from build123d import *

# Parameters (mm, degrees)
F2_SIZE  = 0.79375
F3_R     = 11.1125
F4_DEPTH = 2.3622


with BuildPart() as f1:
    # F0 (on Right) → F1 (revolve)
    with BuildSketch(Plane.YZ):
        Polygon((0, 12.7), (0, 0), (19.05, 0), (19.05, 6.35), (13.396951, 6.35), (5.807927, 12.7), align=None)
    revolve(axis=Axis((0, 9.525, 0), (0, -1, 0)))

    # F2
    f2_edges = [f1.edges().sort_by_distance(p)[0] for p in [
        (0, 0, -12.7),
    ]]
    chamfer(f2_edges, length=F2_SIZE)

    # F3 (on face) → F4 (cut)
    with BuildSketch(Plane.XZ):
        Circle(F3_R)
    extrude(amount=-F4_DEPTH, mode=Mode.SUBTRACT)


solid = f1.part
Read the model definition and answer for the solid it produces. Units are mm, in the model's axes. A direction names the side the tool comes from. Round coordinates to 2 decimals unless told otherwise and drop trailing zeros. Loops run counter-clockwise (first coordinate to the right, second up) from the corner with the lowest first, then second, coordinate; pieces in that order, holes last.
Q1. Each of these flat-tipped pins is pushed along its axis until it touches: pin 1 (3 mm diameter, centred on x = 0, y = 11, fed in from +Z); pin 2 (8 mm diameter, centred on x = -0.5, y = 14, fed in from +Z); pin 3 (3 mm diameter, centred on x = 0, y = 12.5, fed in from +Z); pin 4 (3 mm diameter, centred on y = 14.5, z = -9, fed in from +X). Where does it stop, or does it pass through?
Q2. Section A-A on z = 0 is taken. Write down the section's boundary in (x, y).
Q3. Consider probe 1 along Z at (x, y) = (0, 1.5); probe 2 along Y at (x, z) = (-2, 2.5); probe 3 along Z at (x, y) = (-1.5, 13.5). Determine where each line is inside the solid, lowest interval first.
Q4. Which of the six approach directions +Z, -Z, +X, -X, +Y, -Y give full straight-line access (tool end or side, diameter ignored) to faces 1 (the face through (6.2, 16.18, -1.38)), 2 (the face through (0, 19.05, 0)), 3 (the face through (0, 2.362, 0))?
Q5. Section B-B on x = 0 is taken. Write down the section's boundary in (y, z), and give its area (3 significant figures).
Q6. Section D-D on y = 15.25 is taken. Write down the section's boundary in (x, z), and give its area (3 significant figures).
Q7. Determine the mould class of faces 4 (the face through (10.6, 1.16, 3.34)), 5 (the face through (-2.027, 12.922, 6.436)), 6 (the face through (11, 0, -4)) for opening direction Z: released by +Z, released by -Z, zero draft, split by the parting line, or undercut.
Q8. Section C-C on y = 5.25 is taken. Write down the section's boundary in (x, z), and give its area (3 significant figures).
Output:
1. pin 1: stops at z = 9.61
1. pin 2: stops at z = 9.18
1. pin 3: stops at z = 8.36
1. pin 4: passes through
2. outline: (-12.7, 0.79) - (-11.91, 0) - (-11.11, 0) - (-11.11, 2.36) - (11.11, 2.36) - (11.11, 0) - (11.91, 0) - (12.7, 0.79) - (12.7, 5.81) - (6.35, 13.4) - (6.35, 19.05) - (-6.35, 19.05) - (-6.35, 13.4) - (-12.7, 5.81) - close
3. probe 1: z = -12.7 to -11.11, 11.11 to 12.7
3. probe 2: y = 2.36 to 19.05
3. probe 3: z = -6.17 to 6.17
4. face 1: +Y
4. face 2: +Z, -Z, +X, -X, +Y
4. face 3: -Y
5. outline: (0, -11.91) - (0.79, -12.7) - (5.81, -12.7) - (13.4, -6.35) - (19.05, -6.35) - (19.05, 6.35) - (13.4, 6.35) - (5.81, 12.7) - (0.79, 12.7) - (0, 11.91) - (0, 11.11) - (2.36, 11.11) - (2.36, -11.11) - (0, -11.11) - close
5. area: 311 mm2
6. outline: circle Ø12.7 at (0, 0)
6. area: 127 mm2
7. face 4: undercut
7. face 5: split by the parting line
7. face 6: zero draft
8. outline: circle Ø25.4 at (0, 0)
8. area: 507 mm2
